Design review of the part built by this model. Coordinates are the model's own, in mm. Coordinates: 2 decimals unless noted, no trailing zeros. Write each loop counter-clockwise with the first axis right and the second up, starting at its lowest first coordinate (ties: lowest second). Pieces come first, ordered by that corner, then holes. Notation, with made-up numbers: (67, -20) -> (111, -20) arc R19 cw to (111, 13) -> close; hole circle Ø3 at (49.25, 35). An arc over 180 degrees is marked (long way). Write item = value, one per line. Start each with the question number.
```python
from build123d import *

# Parameters (mm, degrees)
SKETCH1_R           = 4.765
BOSS_EXTRUDE1_DEPTH = 9.525
CHAMFER1_SIZE       = 0.76
SKETCH2_R           = 3.43
CUT_EXTRUDE1_DEPTH  = 9.525


with BuildPart() as part:
    # Sketch1 → Boss-Extrude1 (new body, symmetric)
    with BuildSketch(Plane(origin=(0, 0, 0), x_dir=(0, 0, -1), z_dir=(1, 0, 0))):
        Circle(SKETCH1_R)
    extrude(amount=BOSS_EXTRUDE1_DEPTH, both=True)

    # Chamfer1
    chamfer1_edges = [part.edges().sort_by_distance(p)[0] for p in [
        (-9.525, 0, 4.765),
        (9.525, 0, 4.765),
    ]]
    chamfer(chamfer1_edges, length=CHAMFER1_SIZE)

    # Sketch2 → Cut-Extrude1 (cut, symmetric)
    with BuildSketch(Plane(origin=(0, 0, 0), x_dir=(1, 0, 0), z_dir=(0, 1, 0))):
        with Locations((0, -0.25)):
            Circle(SKETCH2_R)
    extrude(amount=CUT_EXTRUDE1_DEPTH, both=True, mode=Mode.SUBTRACT)


solid = part.part
```
(1) For line 1 (X direction, y = -3, z = 0.25) (3 decimals); line 2 (Z direction, x = -2.5, y = -0.5); line 3 (Z direction, x = -3, y = 2.25), list the stretches that pass through material, from the lowest coordinate up.
(2) Take a section at C-C, the plane x = 0. State the section outline as (y, z) points (3 decimals), then the cut area to 3 significant figures.
(3) Take a section at B-B, the plane z = 0. State the section outline as (x, y) points (3 decimals).
(4) Take a section at A-A, the plane y = 0. State the section outline as (x, z) points (3 decimals).
(5) Take a section at D-D, the plane x = -2. State the section outline as (y, z) points (3 decimals), then the cut area to 3 significant figures.
(6) Mouldability with a two-part tool opening along Z and no side actions: class faces 1 (the face through (9.525, 0, 0)), 2 (the face through (1.844, 0.067, -2.642)), 3 (the face through (0.12, 0.21, 4.76)) as pulls with the +Z half, pulls with the -Z half, needs draft (parallel to the pull), parting line crosses it, or undercut.
(7) For pin 1 Ø4 at (x, z) = (0, 0.25) entering from +Y, flat-tipped, find the tip position at first contact; note if it passes through.
Report:
q1.line_1 = -9.525 to -3.43, 3.43 to 9.525
q1.line_2 = -4.74 to -2.1, 2.6 to 4.74
q1.line_3 = -4.2 to -1.41, 1.91 to 4.2
q2.outline = (-3.549, -3.18) arc R4.765 ccw to (3.549, -3.18) -> close; (-3.027, 3.68) -> (3.027, 3.68) arc R4.765 ccw to start
q2.area = 12.3 mm2
q3.outline = (-9.525, -4.005) -> (-8.765, -4.765) -> (-3.421, -4.765) -> (-3.421, 4.765) -> (-8.765, 4.765) -> (-9.525, 4.005) -> close; (3.421, -4.765) -> (8.765, -4.765) -> (9.525, -4.005) -> (9.525, 4.005) -> (8.765, 4.765) -> (3.421, 4.765) -> close
q4.outline = (-9.525, -4.005) -> (-8.765, -4.765) -> (8.765, -4.765) -> (9.525, -4.005) -> (9.525, 4.005) -> (8.765, 4.765) -> (-8.765, 4.765) -> (-9.525, 4.005) -> close; hole circle Ø6.86 at (0, 0.25)
q5.outline = (-4.034, -2.537) arc R4.765 ccw to (4.034, -2.537) -> close; (-3.672, 3.037) -> (3.672, 3.037) arc R4.765 ccw to start
q5.area = 21.5 mm2
q6.face_1 = needs draft
q6.face_2 = undercut
q6.face_3 = parting line crosses it
q7.pin_1 = through
